Geometry check sheet. Reference: the model listing, model coordinates, mm. A direction names the side the tool comes from. Round coordinates to 2 decimals unless told otherwise and drop trailing zeros. Order: outer loops, then holes, each group sorted by start corner. A loop starts at its lowest first (then second) coordinate and runs counter-clockwise, first axis right, second up. Notation, with made-up numbers: (-17.5, 50.25) -> (-11.5, 50.25) arc R26 ccw to (-11.5, 73.25) -> close; hole circle Ø5 at (71, 70). An arc over 180 degrees is marked (long way). Use a Markdown table: item, result. Add a question column.
Item 1: Set-up check for faces 1 (the cylindrical face through (-29.183, -17.079, 1.932)), 2 (the flat face through (-27, -25.164, 8)), 3 (the flat face through (-27, -13, 10.033)): record each of +Z, -Z, +X, -X, +Y, -Y from which the full face is reachable in a straight line by a thin tool's end or side.
Item 2: Sectioned sample at A-A, the plane y = -14.5. Record the cut outline in (x, z) (3 decimals).
Item 3: Sectioned sample at C-C, the plane x = -18. Record the cut outline in (y, z) (3 decimals).
Item 4: Material ranges on probe 1 along Z at (x, y) = (-19.5, -22) (3 decimals); probe 2 along Z at (x, y) = (-33, -4.5); probe 3 along Y at (x, z) = (-23.5, 11.5), recorded low to high. Write a range as [from, to].
Item 5: Mould release check, pull along Y, two halves, no side actions. Record for faces 4 (the cylindrical face through (-41.987, -10.354, 0.764)), 5 (the cylindrical face through (-26.7, 5.8, 0.7)), 6 (the cylindrical face through (-29.744, -5.759, 2.576)): pulls with the +Y half, pulls with the -Y half, needs draft (parallel to the pull), parting line crosses it, or undercut.
Item 6: Sectioned sample at B-B, the plane x = -22.5. Record the cut outline in (y, z) (3 decimals), and give its area (3 significant figures).
Item 7: Gauge pin test, flat ends, axial feed: pin 1 Ø3 at (x, y) = (-26.84, -18.05) entering from -Z; pin 2 Ø5 at (y, z) = (0, 12.5) entering from -X; pin 3 Ø1.2 at (y, z) = (-14, 15) entering from -X. Record the tip position at first contact, or that the pin passes through.
from build123d import *

# Parameters (mm, degrees)
F0_W     = 31.75
F0_H     = 31.75
F1_DEPTH = 15.875
F3_DEPTH = 25.4
F5_D     = 5.08
F5_DEPTH = 3.81
F5_TIP   = 1.5261859723
F7_D     = 6.096
F7_DEPTH = 5.08
F7_TIP   = 1.8314231668
F8_R     = 6.35
F9_R     = 2.54


with BuildPart() as f1:
    # F0 (on Top) → F1 (new body)
    with BuildSketch(Plane.XY):
        with Locations((-26.8367353499, -9.2885306659)):
            Rectangle(F0_W, F0_H)
    extrude(amount=F1_DEPTH)

    # F2 (on face) → F3 (cut)
    with BuildSketch(Plane.XZ.offset(25.1635306659)):
        Polygon((-20.1692353499, 15.875), (-33.5042353499, 15.875), (-33.5042353499, 14.351), (-36.9967353499, 14.351), (-36.9967353499, 10.033), (-16.6767353499, 10.033), (-16.6767353499, 14.351), (-20.1692353499, 14.351), align=None)
    extrude(amount=-F3_DEPTH, mode=Mode.SUBTRACT)

    # F5
    with Locations(Plane(origin=(0, 0, 0), x_dir=(1, 0, 0), z_dir=(0, 0, -1))):
        with Locations((-26.8367353499, 18.0515306659)):
            Hole(F5_D / 2, depth=F5_DEPTH)
            with Locations((0, 0, -(F5_DEPTH + F5_TIP / 2))):  # 118° drill point
                Cone(0, F5_D / 2, F5_TIP, mode=Mode.SUBTRACT)

    # F7
    with Locations(Plane(origin=(0, 0, 0), x_dir=(1, 0, 0), z_dir=(0, 0, -1))):
        with Locations((-26.8367353499, 4.8435306659)):
            Hole(F7_D / 2, depth=F7_DEPTH)
            with Locations((0, 0, -(F7_DEPTH + F7_TIP / 2))):  # 118° drill point
                Cone(0, F7_D / 2, F7_TIP, mode=Mode.SUBTRACT)

    # F8
    f8_edges = [f1.edges().sort_by_distance(p)[0] for p in [
        (-42.711735, -9.288531, 15.875),
        (-10.961735, -9.288531, 15.875),
    ]]
    fillet(f8_edges, radius=F8_R)

    # F9
    f9_edges = [f1.edges().sort_by_distance(p)[0] for p in [
        (-42.711735, -9.288531, 0),
        (-10.961735, -9.288531, 0),
        (-26.836735, -25.163531, 0),
        (-26.836735, 6.586469, 0),
        (-26.836735, 6.586469, 15.875),
    ]]
    fillet(f9_edges, radius=F9_R)


solid = f1.part
Found:
| question | item | result |
|---|---|---|
| 1 | face 1 | -Z |
| 1 | face 2 | +Z, -Z, +X, -X, -Y |
| 1 | face 3 | -Y |
| 2 | outline | (-42.712, 2.54) arc R2.54 ccw to (-40.172, 0) -> (-13.502, 0) arc R2.54 ccw to (-10.962, 2.54) -> (-10.962, 9.525) arc R6.35 ccw to (-17.312, 15.875) -> (-20.169, 15.875) -> (-20.169, 14.351) -> (-16.677, 14.351) -> (-16.677, 10.033) -> (-36.997, 10.033) -> (-36.997, 14.351) -> (-33.504, 14.351) -> (-33.504, 15.875) -> (-36.362, 15.875) arc R6.35 ccw to (-42.712, 9.525) -> close |
| 3 | outline | (-25.164, 2.54) arc R2.54 ccw to (-22.624, 0) -> (4.046, 0) arc R2.54 ccw to (6.586, 2.54) -> (6.586, 13.335) arc R2.54 ccw to (4.046, 15.875) -> (-25.164, 15.875) -> (-25.164, 14.351) -> (0.236, 14.351) -> (0.236, 10.033) -> (-25.164, 10.033) -> close |
| 4 | probe 1 | z = [0, 10.033], [14.351, 15.875] |
| 4 | probe 2 | z = [0, 10.03] |
| 4 | probe 3 | y = [0.24, 6.59] |
| 5 | face 4 | needs draft |
| 5 | face 5 | pulls with the +Y half |
| 5 | face 6 | undercut |
| 6 | outline | (-25.164, 2.54) arc R2.54 ccw to (-22.624, 0) -> (4.046, 0) arc R2.54 ccw to (6.586, 2.54) -> (6.586, 13.335) arc R2.54 ccw to (4.046, 15.875) -> (0.236, 15.875) -> (0.236, 10.033) -> (-25.164, 10.033) -> close |
| 6 | area | 351 mm2 |
| 7 | pin 1 | stops at z = 4.43 |
| 7 | pin 2 | stops at x = -42.69 |
| 7 | pin 3 | stops at x = -40.43 |
